Design review of the part built by this model. Coordinates are the model's own, in mm. A direction names the side the tool comes from. Give positions to 0.01 mm unless a question says otherwise; leave off trailing zeros. Loops run counter-clockwise (first coordinate to the right, second up) from the corner with the lowest first, then second, coordinate; pieces in that order, holes last. Notation, with made-up numbers: M 42,21.5 L 100,21.5 A16 ccw 100,52.5 Z; hole C 62,11 d5. An arc over 180 degrees is marked long. Use CSV: the item, a comma, the result in double quotes.
from build123d import *

# Parameters (mm, degrees)
BOSS_EXTRUDE3_DEPTH      = 165.1
CUT_EXTRUDE1_DEPTH       = 160.3375
BOSS_EXTRUDE4_DEPTH      = 4.7625
CUT_EXTRUDE2_DEPTH       = 11.176
CUT_EXTRUDE2_DEPTH_BACK  = 387.2865
BOSS_EXTRUDE5_DEPTH      = 365.125
CUT_EXTRUDE3_DEPTH       = 365.125
CUT_EXTRUDE4_DEPTH       = 365.125
BOSS_EXTRUDE6_DEPTH      = 1.27
BOSS_EXTRUDE6_DEPTH_BACK = 216.027
CUT_EXTRUDE5_DEPTH       = 398.907
CUT_EXTRUDE7_DEPTH       = 398.907
CUT_EXTRUDE8_DEPTH       = 216.281
BOSS_EXTRUDE7_DEPTH      = 216.281
CUT_EXTRUDE9_DEPTH       = 216.281
CUT_EXTRUDE10_DEPTH      = 2540


with BuildPart() as part:
    # Sketch13 → Boss-Extrude3 (new body)
    with BuildSketch(Plane.XY):
        Polygon((0, 0), (0, 179.978975516), (35.921024484, 215.9), (329.203975516, 215.9), (365.125, 179.978975516), (365.125, 0), align=None)
    extrude(amount=BOSS_EXTRUDE3_DEPTH)

    # Sketch14 → Cut-Extrude1 (cut)
    with BuildSketch(Plane.XY.offset(165.1)):
        Polygon((4.7625, 0), (4.7625, 177.794773237), (38.105226763, 211.1375), (327.231283425, 211.1375), (360.3625, 178.006283425), (360.3625, 0), align=None)
    extrude(amount=-CUT_EXTRUDE1_DEPTH, mode=Mode.SUBTRACT)

    # Sketch15 → Boss-Extrude4 (add)
    with BuildSketch(Plane.XY.offset(165.1)):
        Polygon((0, 0), (0, 179.978975516), (35.921024484, 215.9), (329.203975516, 215.9), (365.125, 179.978975516), (365.125, 0), align=None)
    extrude(amount=-BOSS_EXTRUDE4_DEPTH)

    # Sketch16 → Cut-Extrude2 (cut, two sides)
    with BuildSketch(Plane(origin=(365.125, 0, 0), x_dir=(0, 0, -1), z_dir=(1, 0, 0))) as cut_extrude2_sk:
        Polygon((-165.1, 179.978975516), (-129.178975516, 215.9), (-165.1, 215.9), align=None)
    extrude(amount=CUT_EXTRUDE2_DEPTH, mode=Mode.SUBTRACT)
    extrude(cut_extrude2_sk.sketch, amount=-CUT_EXTRUDE2_DEPTH_BACK, mode=Mode.SUBTRACT)

    # Sketch17 → Boss-Extrude5 (add)
    with BuildSketch(Plane(origin=(365.125, 0, 0), x_dir=(0, 0, -1), z_dir=(1, 0, 0))):
        Polygon((-165.1, 179.978975516), (-129.178975516, 215.9), (-125.81137947, 212.532403955), (-161.732403955, 176.61137947), align=None)
    extrude(amount=-BOSS_EXTRUDE5_DEPTH)

    # Sketch18 → Cut-Extrude3 (cut)
    with BuildSketch(Plane(origin=(0, 0, 0), x_dir=(-1, 0, 0), z_dir=(0, 0, -1))):
        Polygon((-365.125, 179.978975516), (-329.203975516, 215.9), (-365.125, 215.9), align=None)
        Polygon((-35.921024484, 215.9), (0, 215.9), (0, 179.978975516), align=None)
    extrude(amount=-CUT_EXTRUDE3_DEPTH, mode=Mode.SUBTRACT)

    # Sketch19 → Cut-Extrude4 (cut)
    with BuildSketch(Plane(origin=(0, 215.9, 0), x_dir=(1, 0, 0), z_dir=(0, 1, 0))):
        Polygon((0, -129.178975516), (35.921024484, -165.1), (0, -165.1), align=None)
    extrude(amount=-CUT_EXTRUDE4_DEPTH, mode=Mode.SUBTRACT)

    # Sketch20 → Boss-Extrude6 (add, two sides)
    with BuildSketch(Plane(origin=(0, 215.9, 0), x_dir=(1, 0, 0), z_dir=(0, 1, 0))) as boss_extrude6_sk:
        Polygon((0, -129.178975516), (35.921024484, -165.1), (39.28862053, -161.732403955), (3.367596045, -125.81137947), align=None)
    extrude(amount=BOSS_EXTRUDE6_DEPTH)
    extrude(boss_extrude6_sk.sketch, amount=-BOSS_EXTRUDE6_DEPTH_BACK)

    # Sketch21 → Cut-Extrude5 (cut)
    with BuildSketch(Plane(origin=(365.125, 0, 0), x_dir=(0, 0, -1), z_dir=(1, 0, 0))):
        Polygon((-165.1, 179.978975516), (-129.178975516, 215.9), (-125.060291361, 215.9), (-125.060291361, 220.601518186), (-193.24025866, 220.601518186), (-185.719207112, 179.978975516), align=None)
    extrude(amount=-CUT_EXTRUDE5_DEPTH, mode=Mode.SUBTRACT)

    # Sketch22 → Cut-Extrude7 (cut)
    with BuildSketch(Plane(origin=(0, 0, 0), x_dir=(-1, 0, 0), z_dir=(0, 0, -1))):
        Polygon((0, 179.978975516), (-35.921024484, 215.9), (-15.545950188, 236.275074296), (20.375074296, 200.354049812), align=None)
    extrude(amount=-CUT_EXTRUDE7_DEPTH, mode=Mode.SUBTRACT)

    # Sketch24 → Cut-Extrude8 (cut)
    with BuildSketch(Plane(origin=(0, 215.9, 0), x_dir=(1, 0, 0), z_dir=(0, 1, 0))):
        Polygon((329.203975516, -165.1), (365.125, -129.178975516), (387.404902752, -151.458878267), (351.483878267, -187.379902752), align=None)
    extrude(amount=-CUT_EXTRUDE8_DEPTH, mode=Mode.SUBTRACT)

    # Sketch25 → Boss-Extrude7 (add)
    with BuildSketch(Plane(origin=(0, 215.9, 0), x_dir=(1, 0, 0), z_dir=(0, 1, 0))):
        Polygon((329.203975516, -165.1), (365.125, -129.178975516), (361.757403955, -125.81137947), (325.83637947, -161.732403955), align=None)
    extrude(amount=-BOSS_EXTRUDE7_DEPTH)

    # Sketch26 → Cut-Extrude9 (cut)
    with BuildSketch(Plane(origin=(0, 0, 0), x_dir=(-1, 0, 0), z_dir=(0, 0, -1))):
        Polygon((-365.125, 179.978975516), (-329.203975516, 215.9), (-357.158082667, 243.854107151), (-393.079107151, 207.933082667), align=None)
    extrude(amount=-CUT_EXTRUDE9_DEPTH, mode=Mode.SUBTRACT)

    # Sketch27 → Cut-Extrude10 (cut)
    with BuildSketch(Plane.ZY):
        Polygon((129.178975516, 215.9), (165.1, 179.978975516), (185.560673149, 200.439648664), (149.639648664, 236.360673149), align=None)
    extrude(amount=-CUT_EXTRUDE10_DEPTH, mode=Mode.SUBTRACT)


solid = part.part
(1) Machinability: for faces 5 (the flat face through (185, 109, 0)), 6 (the flat face through (184.872, 194.804, 143.54)), which of the approach directions +Z, -Z, +X, -X, +Y, -Y give a long, thin tool a straight path to every point of the face, cutting with its end or side? Answer none if there is none.
A:
face 5,"-Z, +X, -X, +Y, -Y"
face 6,"-Y"
(2) Wall thickness on line 1 along X through (y, z) = (135, 22) (1 decimal); line 2 along Z through (x, y) = (159.5, 84); line 3 along Y through (x, z) = (247, 62): over which ranges is each line inside the solid? List them lowest first. Write a range as [from, to].
A:
line 1,"[0, 4.8], [360.4, 365.1]"
line 2,"[0, 4.76], [160.34, 165.1]"
line 3,"[211.14, 215.9]"
(3) We need section C-C on x = 114. State the section outline as (y, z) points.
A:
outline,"M 0,0 L 215.9,0 L 215.9,129.18 L 179.98,165.1 L 0,165.1 L 0,160.34 L 178.01,160.34 L 211.14,127.21 L 211.14,4.76 L 0,4.76 Z"
(4) We need section B-B on z = 14. State the section outline as (x, y) points (1 decimal).
A:
outline,"M 0,0 L 4.8,0 L 4.8,177.8 L 38.1,211.1 L 327.2,211.1 L 360.4,178 L 360.4,0 L 365.1,0 L 365.1,180 L 329.2,215.9 L 35.9,215.9 L 0,180 Z"
(5) The part is to be moulded in two halves that separate along Z. For faces 1 (the flat face through (17.71, 100.29, 146.89)), 2 (the flat face through (181, 211.138, 67)), 3 (the flat face through (17.71, 197.69, 72.54)), 4 (the flat face through (21.2, 194.23, 75.29)), say which applies: released by +Z, released by -Z, zero draft, split by the parting line, or undercut.
A:
face 1,"released by +Z"
face 2,"undercut"
face 3,"zero draft"
face 4,"undercut"
(6) We need section D-D on z = 134. State the section outline as (x, y) points (3 decimals).
A:
outline,"M 4.821,-0.127 L 11.556,-0.127 L 11.556,184.588 L 31.312,204.344 L 334.025,204.344 L 353.569,184.8 L 353.569,-0.381 L 360.304,-0.381 L 360.304,184.8 L 334.025,211.079 L 31.1,211.079 L 4.821,184.8 Z"
(7) Clearance check with flat-ended pins moving along their axes: P1, Ø8, axis at x = 303, z = 105, coming from the -Y side; P2, Ø2.5, axis at x = 234.5, z = 163, coming from the -Y side; P3, Ø12, axis at x = 20, z = 140, coming from the -Y side. State where each tip first meets the part, or that it passes through.
A:
P1,"y = 211.14"
P2,"y = 0"
P3,"y = -0.13"
(8) We need section A-A on y = 113. State the section outline as (x, z) points (1 decimal).
A:
outline,"M 0,0 L 365.1,0 L 365.1,129.2 L 329.2,165.1 L 35.9,165.1 L 0,129.2 Z; hole M 4.8,4.8 L 360.4,4.8 L 360.4,127.2 L 327.2,160.3 L 37.9,160.3 L 4.8,127.2 Z"
